Check sheet for the modelled part. Datum: model origin and axes. Units: mm. A direction names the side the tool comes from. Coordinates: 2 decimals unless noted, no trailing zeros. Write each loop counter-clockwise with the first axis right and the second up, starting at its lowest first coordinate (ties: lowest second). Pieces come first, ordered by that corner, then holes. Notation, with made-up numbers: M -17.5,-29 L 17.5,-29 A21 ccw 17.5,-22 Z; hole C 1.25,17.5 d6. An arc over 180 degrees is marked long. Answer as CSV lines item,"result". Start each with the question number.
Q1. Sectioned sample at C-C, the plane z = 41.5. Record the cut outline in (x, y), then the cut area to 3 significant figures.
Q2. Sectioned sample at D-D, the plane x = 234. Record the cut outline in (y, z), then the cut area to 3 significant figures.
Q3. Access from +Z, -Z, +X, -X, +Y, -Y to the whole of each face (thin tool, end or side, straight path). Record for faces 5 (the flat face through (128.5, -24, 74.7)), 6 (the flat face through (160, 101.6, 73)).
Q4. Depth check by flat-ended pin: pin 1 Ø1.5 at (y, z) = (-47, 99.5) entering from -X; pin 2 Ø5 at (x, y) = (191, 73.5) entering from +Z. Enter the tip coordinate at first touch or a pass-through.
Q5. Thickness scan on line 1 along Z through (x, y) = (10, -14); line 2 along Z through (x, y) = (92.5, -28.5); line 3 along Z through (x, y) = (125, 60). Record the ranges inside material, lowest first. Write a range as from..to.
Q6. Mould release check, pull along Z, two halves, no side actions. Record for faces 1 (the flat face through (160, -101.6, 73)), 2 (the flat face through (77, -1, 50.8)), 3 (the flat face through (125, -1, 0)), 4 (the cylindrical face through (156.473, -8.259, 98.238)): pulls with the +Z half, pulls with the -Z half, needs draft (parallel to the pull), parting line crosses it, or undercut.
Q7. Sectioned sample at B-B, the plane y = -3.5. Record the cut outline in (x, z), then the cut area to 3 significant figures.
Q8. Sectioned sample at A-A, the plane y = -82. Record the cut outline in (x, z), then the cut area to 3 significant figures.
from build123d import *

# Parameters (mm, degrees)
F1_DEPTH      = 101.6
F3_DEPTH      = 50.801
F5_R          = 38.1
F6_DEPTH      = 101.6
F6_DEPTH_BACK = 101.6


with BuildPart() as f1:
    # F0 (on Front) → F1 (new body, symmetric)
    with BuildSketch(Plane.XZ):
        Polygon((0, 50.8), (0, 0), (254, 0), (254, 50.8), (119.296158184, 185.503841816), (68.496158184, 134.703841816), (152.4, 50.8), align=None)
    extrude(amount=F1_DEPTH, both=True)

    # F2 (on face) → F3 (cut, through all)
    with BuildSketch(Plane.XY.offset(50.8)):
        Polygon((76.2, 101.6), (0, 101.6), (0, 50.8), align=None)
        Polygon((76.2, -101.6), (0, -50.8), (0, -101.6), align=None)
    extrude(amount=-F3_DEPTH, mode=Mode.SUBTRACT)

    # F5 (on offset) → F6 (cut, two sides)
    with BuildSketch(Plane(origin=(170.3605122421, 0, 170.3605122421), x_dir=(0, 1, 0), z_dir=(0.7071067812, 0, 0.7071067812))) as f6_sk:
        with Locations((0, -3.9840979371)):
            Circle(F5_R)
    extrude(amount=F6_DEPTH, mode=Mode.SUBTRACT)
    extrude(f6_sk.sketch, amount=-F6_DEPTH_BACK, mode=Mode.SUBTRACT)


solid = f1.part
Output:
1,outline,"M 0,-50.8 L 76.2,-101.6 L 254,-101.6 L 254,101.6 L 76.2,101.6 L 0,50.8 Z"
1,area,"47,700 mm^2"
2,outline,"M -101.6,0 L 101.6,0 L 101.6,70.8 L -101.6,70.8 Z"
2,area,"14,400 mm^2"
3,face 5,"-X, +Y, -Y"
3,face 6,"+Z, -Z, +X, -X, +Y"
4,pin 1,"stops at x = 102.95"
4,pin 2,"stops at z = 116.3"
5,line 1,"z = 0..50.8"
5,line 2,"z = 0..50.8, 122.62..158.71"
5,line 3,"z = 0..50.8, 78.2..179.8"
6,face 1,"needs draft"
6,face 2,"undercut"
6,face 3,"pulls with the -Z half"
6,face 4,"undercut"
7,outline,"M 0,0 L 254,0 L 254,50.8 L 182.04,122.76 L 131.24,71.96 L 152.4,50.8 L 0,50.8 Z; M 68.5,134.7 L 77.59,125.61 L 128.39,176.41 L 119.3,185.5 Z"
7,area,"18,600 mm^2"
8,outline,"M 46.8,0 L 254,0 L 254,50.8 L 119.3,185.5 L 68.5,134.7 L 152.4,50.8 L 46.8,50.8 Z"
8,area,"21,600 mm^2"
